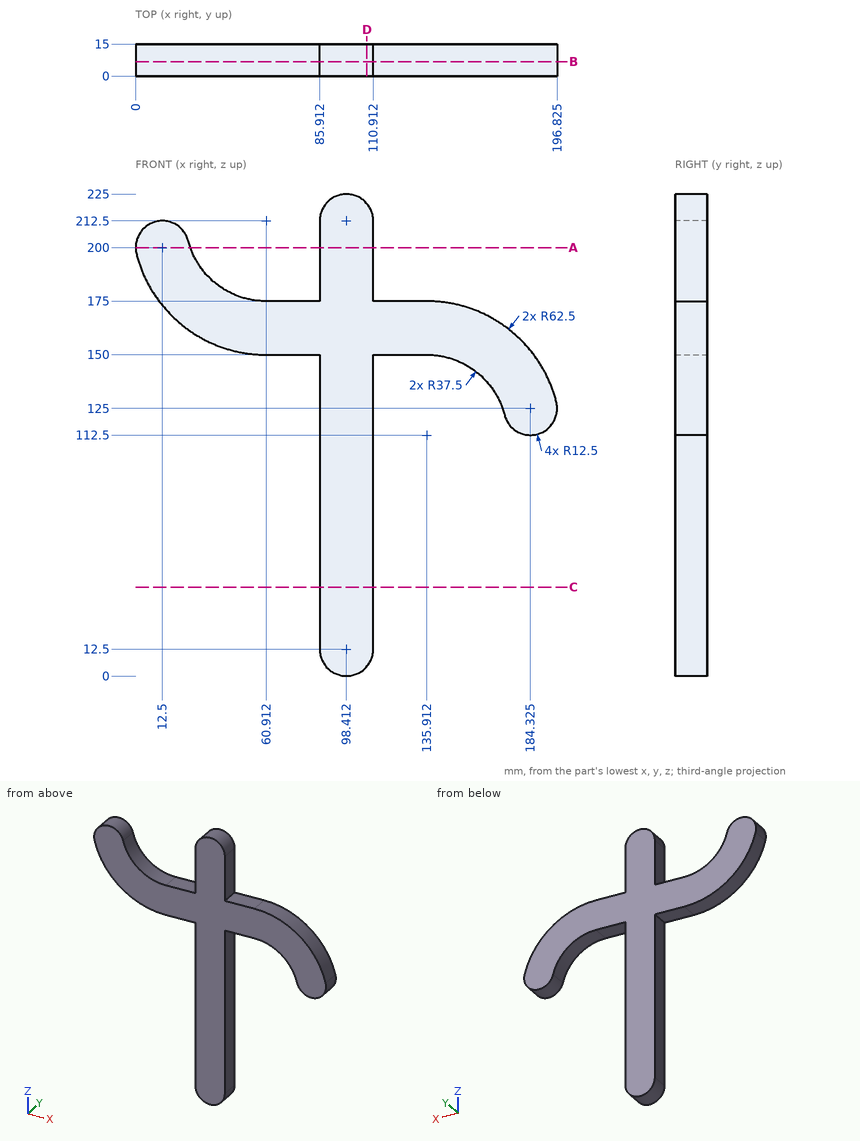
Could you check a few things on this drawing? It's one solid part, dimensions in mm from its lowest x, y, z. Coordinates: 2 decimals unless noted, no trailing zeros. Order: outer loops, then holes, each group sorted by start corner. A loop starts at its lowest first (then second) coordinate and runs counter-clockwise, first axis right, second up. Notation, with made-up numbers: (-34, 74.5) - (-9, 74.5) arc R18 ccw to (-9, 95.5) - close; hole circle Ø10 at (-28, 7.25). An arc over 180 degrees is marked (long way). Answer as a JSON object with one key per item and string values. Group by question number.
Q1. Imagine slicing it at A-A (z = 200). Please give me the cut outline in (x, y).
Q2. Will these pins go through, and if not, where does the flat tip stop? P1, Ø2, axis at y = 13.5, z = 80.5, coming from the +X side; P2, Ø7.5, axis at x = 119.5, y = 7.5, coming from the -Z side; P3, Ø2, axis at x = 74, y = 2, coming from the +Z side.
Q3. Imagine slicing it at C-C (z = 41.5). Please give me the cut outline in (x, y), and give its area (3 significant figures).
Q4. Imagine slicing it at D-D (x = 108). Please give me the cut outline in (y, z).
Q5. Imagine slicing it at B-B (y = 6.75). Please give me the cut outline in (x, z) (1 decimal), and give its area (3 significant figures).
Q6. I need wall thicknesses on line 1 (Z direction, x = 133.5, y = 9); line 2 (X direction, y = 11.5, z = 27); line 3 (X direction, y = 2.25, z = 202). Which ranges of each line are inside material? Lowest first, please. Write a range as from..to.
Determined:
{
 "1": {"outline": "(0, 0) - (25.56, 0) - (25.56, 15) - (0, 15) - close; (85.91, 0) - (110.91, 0) - (110.91, 15) - (85.91, 15) - close"},
 "2": {"P1": "stops at x = 110.91", "P2": "stops at z = 150", "P3": "stops at z = 175"},
 "3": {"outline": "(85.91, 0) - (110.91, 0) - (110.91, 15) - (85.91, 15) - close", "area": "375 mm2"},
 "4": {"outline": "(0, 4.48) - (15, 4.48) - (15, 220.52) - (0, 220.52) - close"},
 "5": {"outline": "(0.4, 196.9) arc R62.5 ccw to (60.9, 150) - (85.9, 150) - (85.9, 12.5) arc R12.5 ccw to (110.9, 12.5) - (110.9, 150) - (135.9, 150) arc R37.5 cw to (172.2, 121.9) arc R12.5 ccw to (196.4, 128.1) arc R62.5 ccw to (135.9, 175) - (110.9, 175) - (110.9, 212.5) arc R12.5 ccw to (85.9, 212.5) - (85.9, 175) - (60.9, 175) arc R37.5 cw to (24.6, 203.1) arc R12.5 ccw to start", "area": "10,500 mm2"},
 "6": {"line 1": "z = 150..175", "line 2": "x = 85.91..110.91", "line 3": "x = 0.16..24.91, 85.91..110.91"}
}
